The listing builds one solid part. Answer for the finished solid, in the listing's coordinates (mm). A direction names the side the tool comes from. Coordinates: 2 decimals unless noted, no trailing zeros. Loops run counter-clockwise (first coordinate to the right, second up) from the corner with the lowest first, then second, coordinate; pieces in that order, holes last. Notation, with made-up numbers: M -7.5,74.5 L 1.5,74.5 A21 ccw 1.5,89.5 Z; hole C 41,-8.5 d4. An arc over 180 degrees is marked long. Return JSON: item names as keys, results as strings. Group by question number.
1. Section B-B (y = 11.5) is taken. Write down the section's boundary in (x, z).
2. Which of the six approach directions +Z, -Z, +X, -X, +Y, -Y give full straight-line access (tool end or side, diameter ignored) to faces 1 (the face through (-8.496, 39.087, 4.93)), 2 (the face through (-5.1, 38.16, 5.56)), 3 (the face through (50, 24.5, 0.2))?
3. Straight lines are drawn through the part: L1, parallel to X at y = 43.5, z = 28.5; L2, parallel to Z at x = 28, y = 32; L3, parallel to Y at x = 7, z = 21. For each, find the intervals that lie inside material, in ascending order. Write a range as from..to.
4. Section C-C (z = 9) is taken. Write down the section's boundary in (x, y), then the cut area to 3 significant figures.
5. The mould has two halves that part along Y. Classify faces 4 (the face through (-38.91, 9.27, 4.93)), 5 (the face through (31.39, 43.21, 18.25)), 6 (the face through (-38, 9, 10)), 7 (the face through (-3.164, 48.502, 18.252)): pulls with the +Y half, pulls with the -Y half, needs draft (parallel to the pull), parting line crosses it, or undercut.
6. Section D-D (x = 40) is taken. Write down the section's boundary in (y, z).
7. Given P1, Ø6, axis at y = 26, z = 28, coming from the -X side; P2, Ø0.7, axis at x = -7.5, y = 39, coming from the +Z side; P3, Ø1.5, axis at y = 43.5, z = 25, coming from the +X side, each flat-ended and moving along its own axis, determine where each tip first touches the part or whether it passes through.
8. Section A-A (z = 21) is taken. Write down the section's boundary in (x, y).
```python
from build123d import *

# Parameters (mm, degrees)
PAD_DEPTH         = 10
POCKET_DEPTH      = 9
PAD001_DEPTH      = 35
PAD001_DEPTH_BACK = 1
SKETCH007_R       = 12.8
POCKET001_DEPTH   = 67.6190458501
SKETCH004_R       = 11.2
POCKET002_DEPTH   = 77.1582330742


with BuildPart() as part:
    # Sketch → Pad (new body)
    with BuildSketch(Plane.XY):
        with BuildLine():
            ThreePointArc((30, 0), (0, 30), (-30, 0))
            Line((-40, 0), (-30, 0))
            ThreePointArc((0, 40), (-28.2842712475, 28.2842712475), (-40, 0))
            Line((0, 40), (50, 40))
            Line((50, 40), (50, 0))
            Line((30, 0), (50, 0))
        make_face()
    extrude(amount=PAD_DEPTH)

    # Sketch002 → Pocket (cut)
    with BuildSketch(Plane.XY.offset(10)):
        with BuildLine():
            ThreePointArc((0, 38.5), (-27.2236110757, 27.2236110757), (-38.5, 0))
            Line((65, -6.5), (-38.5, 0))
            Line((65, 38.5), (65, -6.5))
            Line((0, 38.5), (65, 38.5))
        make_face()
    extrude(amount=-POCKET_DEPTH, mode=Mode.SUBTRACT)

    # Sketch003 → Pad001 (new body, two sides)
    with BuildSketch(Plane.XY.offset(1)) as pad001_sk:
        Polygon((-0.3768292053, 58.2286851346), (-6.0296340472, 38.5), (29.9497560282, 38.5), (32.8734730754, 48.0630475596), align=None)
        Polygon((-16.6802067695, 44.7702775725), (-41.1936289493, 24.2010740626), (-34.7657528524, 16.5406296314), (-10.2523306726, 37.1098331414), align=None)
    extrude(amount=PAD001_DEPTH)
    extrude(pad001_sk.sketch, amount=-PAD001_DEPTH_BACK)

    # Sketch007 → Pocket001 (cut, through all)
    with BuildSketch(Plane(origin=(16.248321935, 53.1458663471, 0), x_dir=(-0.956304756, 0.2923717047, 0), z_dir=(0.2923717047, 0.956304756, 0))):
        with Locations((0, 36)):
            Circle(SKETCH007_R)
    extrude(amount=-POCKET001_DEPTH, mode=Mode.SUBTRACT)

    # Sketch004 → Pocket002 (cut, through all)
    with BuildSketch(Plane(origin=(-28.9369178594, 34.4856758176, 0), x_dir=(-0.7660444431, -0.6427876097, 0), z_dir=(-0.6427876097, 0.7660444431, 0))):
        with Locations((0, 36)):
            Circle(SKETCH004_R)
    extrude(amount=-POCKET002_DEPTH, mode=Mode.SUBTRACT)


solid = part.part
```
Worked out:
{
 "1": {"outline": "M -38.31,0 L -27.71,0 L -27.71,1 L -36.74,1 L -36.74,10 L -38.31,10 Z; M 27.71,0 L 50,0 L 50,1 L 27.71,1 Z"},
 "2": {"face 1": "+Z, -Z, +Y", "face 2": "+Z, +X, -Y", "face 3": "+Z, -Z, +X, +Y, -Y"},
 "3": {"L1": "-18.19..-15.61, -4.6..2.45, 24.15..31.48", "L2": "0..1", "L3": "38.5..55.97"},
 "4": {"outline": "M -41.19,24.2 L -35.82,17.8 A40 ccw -40,0 L -38.5,0 A38.5 cw -34.77,16.54 L -10.25,37.11 A38.5 cw 0,38.5 L 50,38.5 L 50,40 L 30.41,40 L 32.87,48.06 L -0.38,58.23 L -5.72,39.59 A40 ccw -11.31,38.37 L -16.68,44.77 Z", "area": "914 mm^2"},
 "5": {"face 4": "undercut", "face 5": "undercut", "face 6": "needs draft", "face 7": "pulls with the +Y half"},
 "6": {"outline": "M 0,0 L 40,0 L 40,10 L 38.5,10 L 38.5,1 L 0,1 Z"},
 "7": {"P1": "x = -41.19", "P2": "z = 10", "P3": "x = 31.71"},
 "8": {"outline": "M -41.19,24.2 L -34.77,16.54 L -10.25,37.11 L -16.68,44.77 Z; M -6.03,38.5 L 29.95,38.5 L 32.87,48.06 L -0.38,58.23 Z"}
}
